Design review of the part built by this model. Coordinates are the model's own, in mm. Coordinates: 2 decimals unless noted, no trailing zeros. Loops run counter-clockwise (first coordinate to the right, second up) from the corner with the lowest first, then second, coordinate; pieces in that order, holes last. Notation, with made-up numbers: M -33.5,46.5 L -2.5,46.5 A28 cw -2.5,85.5 Z; hole C 66.5,-6.75 d5. An arc over 180 degrees is marked long. Put each result on its own line as item: value. Start each with the question number.
(1) The part is to be moulded in two halves that separate along Y. For faces 1 (the cylindrical face through (-0.867, -3.905, -0.105)), 2 (the flat face through (3, -3, 7.5)), 3 (the cylindrical face through (-7.493, 0.33, 0.098)), say which applies: +Y half, -Y half, draft (parallel to the pull), parting line (faces both ways), or undercut.
(2) Take a section at A-A, the plane x = 0. Give the boundary of the cut face in (y, z).
(3) Take a section at C-C, the plane z = 4.5. Give the boundary of the cut face in (x, y), then the cut area to 3 significant figures.
(4) For probe 1 along Y at (x, z) = (0, -0.5); probe 2 along X at (y, z) = (-1, -4.5); probe 3 along X at (y, z) = (-1.5, -3), list the stretches that pass through material, from the lowest coordinate up. Write a range as [from, to].
(5) Clearance check with flat-ended pins moving along their axes: pin 1 (6 mm diameter, centred on y = 3.5, z = -5.5, fed in from +X); pin 2 (5 mm diameter, centred on x = 1, z = 3, fed in from +Y); pin 3 (4 mm diameter, centred on x = -6, z = 2, fed in from +Y). State where each tip first meets the part, or that it passes through.
```python
from build123d import *

# Parameters (mm, degrees)
SKETCH_1_R      = 7.5
SKETCH_1_R_2    = 4
EXTRUDE_1_DEPTH = 7.5
CHAMFER_1_SIZE  = 0.5
CHAMFER_2_SIZE  = 0.5


with BuildPart() as part:
    # 草图1 → 凸台-拉伸1 (new, symmetric)
    with BuildSketch(Plane.XY):
        Circle(SKETCH_1_R)
        Circle(SKETCH_1_R_2, mode=Mode.SUBTRACT)
    extrude(amount=EXTRUDE_1_DEPTH, both=True)

    # 倒角1
    chamfer_1_edges = [part.edges().sort_by_distance(p)[0] for p in [
        (-7.5, 0, -7.5),
    ]]
    chamfer(chamfer_1_edges, length=CHAMFER_1_SIZE)

    # 倒角2
    chamfer_2_edges = [part.edges().sort_by_distance(p)[0] for p in [
        (-7.5, 0, 7.5),
    ]]
    chamfer(chamfer_2_edges, length=CHAMFER_2_SIZE)


solid = part.part
```
Computed values:
1. face 1: undercut
1. face 2: draft
1. face 3: parting line
2. outline: M -7.5,-7 L -7,-7.5 L -4,-7.5 L -4,7.5 L -7,7.5 L -7.5,7 Z; M 4,-7.5 L 7,-7.5 L 7.5,-7 L 7.5,7 L 7,7.5 L 4,7.5 Z
3. outline: C 0,0 d15; hole C 0,0 d8
3. area: 126 mm^2
4. probe 1: y = [-7.5, -4], [4, 7.5]
4. probe 2: x = [-7.43, -3.87], [3.87, 7.43]
4. probe 3: x = [-7.35, -3.71], [3.71, 7.35]
5. pin 1: stops at x = 7.48
5. pin 2: stops at y = 7.5
5. pin 3: stops at y = 6.34
